from build123d import *

# Parameters (mm, degrees)
SKETCH_1_R          = 1.7
EXTRUDE_1_DEPTH     = 3
EXTRUDE_2_DEPTH     = 13
EXTRUDE_3_DEPTH     = 18
SKETCH_5_R          = 1.8
CUT_EXTRUDE_1_DEPTH = 34
FILLET_1_R          = 2
CHAMFER_1_SIZE      = 1
FILLET_2_R          = 2


with BuildPart() as part:
    # Эскиз1 → Бобышка-Вытянуть1 (new body)
    with BuildSketch(Plane.XY):
        with BuildLine():
            Line((3.746141591, -1.402292116), (44.253858409, -1.402292116))
            ThreePointArc((44.253858409, -1.402292116), (51.28703274, -2.279345469), (48, 4))
            Line((48, 4), (44.253858409, 7))
            Line((44.253858409, 7), (3.746141591, 7))
            Line((3.746141591, 7), (0, 4))
            ThreePointArc((0, 4), (-3.28703274, -2.279345469), (3.746141591, -1.402292116))
        make_face()
        Circle(SKETCH_1_R, mode=Mode.SUBTRACT)
        with Locations((48, 0)):
            Circle(SKETCH_1_R, mode=Mode.SUBTRACT)
    extrude(amount=EXTRUDE_1_DEPTH)

    # Эскиз2 → Бобышка-Вытянуть2 (add)
    with BuildSketch(Plane.XY.offset(3)):
        Polygon((0, 4), (48, 4), (44.253858409, 7), (3.746141591, 7), align=None)
    extrude(amount=EXTRUDE_2_DEPTH)

    # Эскиз4 → Бобышка-Вытянуть3 (add)
    with BuildSketch(Plane(origin=(0, 7, 0), x_dir=(1, 0, 0), z_dir=(0, 1, 0))):
        Polygon((11, -13), (14, -13), (14, -8), (14, -3), (11, -3), align=None)
        Polygon((34, -8), (34, -3), (37, -3), (37, -13), (34, -13), align=None)
    extrude(amount=EXTRUDE_3_DEPTH)

    # Эскиз5 → Вырез-Вытянуть1 (cut)
    with BuildSketch(Plane.ZY.offset(-11)):
        with Locations(Location((8, 17, 0), (0, 0, 270))):
            Circle(SKETCH_5_R)
    extrude(amount=-CUT_EXTRUDE_1_DEPTH, mode=Mode.SUBTRACT)

    # Скругление1
    fillet_1_edges = [part.edges().sort_by_distance(p)[0] for p in [
        (12.5, 7, 13),
        (14, 7, 8),
        (12.5, 7, 3),
        (11, 7, 8),
        (12.5, 25, 13),
        (12.5, 25, 3),
        (35.5, 25, 13),
        (35.5, 25, 3),
        (34, 7, 8),
        (35.5, 7, 3),
        (37, 7, 8),
        (35.5, 7, 13),
    ]]
    fillet(fillet_1_edges, radius=FILLET_1_R)

    # Фаска1
    # the kernel refuses this chamfer: 1 mm, written as the material it adds along each edge
    with BuildSketch(Plane(origin=(-2.571682988, 4, 3), x_dir=(0, 0.027495876610586053, 0.9996219169112968), z_dir=(1, 0, 0))) as chamfer_1_piece_1_section:
        Polygon((CHAMFER_1_SIZE * 0.999621916911, CHAMFER_1_SIZE * 0.0274958766106), (-CHAMFER_1_SIZE * 0.0274958766106, CHAMFER_1_SIZE * 0.999621916911), (0, 0), align=None)
    chamfer_1_piece_1 = extrude(amount=53.143365976, mode=Mode.PRIVATE)
    chamfer_1_piece_1 = split(chamfer_1_piece_1, bisect_by=Plane(origin=(19.332961003, 26.957252121, 3.279224906), z_dir=(-0.6250871381508221, -0.7805549754619563, 0)), keep=Keep.TOP, mode=Mode.PRIVATE)
    chamfer_1_piece_1 = split(chamfer_1_piece_1, bisect_by=Plane(origin=(0.14685454, 4.117604636, 3.279224906), z_dir=(0.625087138150823, -0.7805549754619556, 0)), keep=Keep.TOP, mode=Mode.PRIVATE)
    add(chamfer_1_piece_1)

    # Скругление2
    fillet_2_edges = [part.edges().sort_by_distance(p)[0] for p in [
        (0, 4, 1.5),
        (48, 4, 1.5),
        (44.253858409, -1.402292116, 1.5),
        (3.746141591, -1.402292116, 1.5),
    ]]
    fillet(fillet_2_edges, radius=FILLET_2_R)


solid = part.part
Read the model definition and answer for the solid it produces. Units are mm, in the model's axes. A direction names the side the tool comes from. Coordinates: 2 decimals unless noted, no trailing zeros. Order: outer loops, then holes, each group sorted by start corner. A loop starts at its lowest first (then second) coordinate and runs counter-clockwise, first axis right, second up. Notation, with made-up numbers: (60, 48) -> (84, 48) arc R29 ccw to (84, 74) -> close; hole circle Ø6 at (59, 12). An arc over 180 degrees is marked (long way). Answer as a JSON object with one key per item and string values.
1) The mould has two halves that part along X. Classify faces 1 (the face through (35.48, 24.4, 12.43)), 2 (the face through (44, -1.64, 1.52)), 3 (the face through (37.6, 7.57, 8.1)): released by +X, released by -X, zero draft, split by the parting line, or undercut.
Model answer:
{"face 1": "zero draft", "face 2": "undercut", "face 3": "released by +X"}
2) A cutting plane is placed at B-B, the plane y = 14.5. Determine the outline of the cut face in (x, z), plus the area to 3 significant figures.
Model answer:
{"outline": "(11, 3) -> (14, 3) -> (14, 13) -> (11, 13) -> close; (34, 3) -> (37, 3) -> (37, 13) -> (34, 13) -> close", "area": "60.0 mm²"}
3) Each of these flat-tipped pins is pushed along its axis until it touches: pin 1 (3.5 mm diameter, centred on x = 35, y = 18.5, fed in from -Z); pin 2 (4 mm diameter, centred on x = 4.5, z = 7.5, fed in from +Y); pin 3 (2 mm diameter, centred on y = 17, z = 8, fed in from +X); pin 4 (4 mm diameter, centred on x = 35.5, y = 21.5, fed in from +Z). Where does it stop, or does it pass through?
Model answer:
{"pin 1": "stops at z = 3", "pin 2": "stops at y = 7", "pin 3": "passes through", "pin 4": "stops at z = 13"}
4) A cutting plane is placed at A-A, the plane z = 8. Determine the outline of the cut face in (x, y).
Model answer:
{"outline": "(0, 4) -> (48, 4) -> (44.25, 7) -> (39, 7) arc R2 cw to (37, 9) -> (37, 15.2) -> (34, 15.2) -> (34, 9) arc R2 cw to (32, 7) -> (16, 7) arc R2 cw to (14, 9) -> (14, 15.2) -> (11, 15.2) -> (11, 9) arc R2 cw to (9, 7) -> (3.75, 7) -> close; (11, 18.8) -> (14, 18.8) -> (14, 25) -> (11, 25) -> close; (34, 18.8) -> (37, 18.8) -> (37, 25) -> (34, 25) -> close"}
5) A tool of negligible diameter and unlimited length cuts with its end or side. For faces 4 (the face through (24, 4, 10)), 5 (the face through (4.024, -1.626, 1.521)), 6 (the face through (35, 16, 3)), 7 (the face through (12, 16, 13)), 8 (the face through (-0.37, -1.66, 1.48)), from which of +Z, -Z, +X, -X, +Y, -Y can it reach the whole face along a straight path? Write none if from no direction.
Model answer:
{"face 4": "+Z, +X, -X, -Y", "face 5": "+Z, -Z, -Y", "face 6": "-Z, +X, -X, +Y", "face 7": "+Z, +X, -X, +Y", "face 8": "+Z, -Z"}
6) Consider line 1 along X through (y, z) = (19, 3.5); line 2 along Z through (x, y) = (6, 1.5); line 3 along Z through (x, y) = (12.1, 17). Determine where each line is inside the solid, lowest interval first. Write a range as from..to.
Model answer:
{"line 1": "x = 11..14, 34..37", "line 2": "z = 0..3", "line 3": "z = 3..6.2, 9.8..13"}
7) A cutting plane is placed at D-D, the plane x = 31. Determine the outline of the cut face in (y, z).
Model answer:
{"outline": "(-1.4, 0) -> (7, 0) -> (7, 16) -> (4, 16) -> (4, 4) -> (3, 3) -> (-1.4, 3) -> close"}
8) A cutting plane is placed at C-C, the plane y = 18.25. Determine the outline of the cut face in (x, z), plus the area to 3 significant figures.
Model answer:
{"outline": "(11, 3) -> (14, 3) -> (14, 6.7) -> (11, 6.7) -> close; (11, 9.3) -> (14, 9.3) -> (14, 13) -> (11, 13) -> close; (34, 3) -> (37, 3) -> (37, 6.7) -> (34, 6.7) -> close; (34, 9.3) -> (37, 9.3) -> (37, 13) -> (34, 13) -> close", "area": "44.5 mm²"}
